Can you work these out from the model? Positions are in its coordinate system, mm. A direction names the side the tool comes from. Give positions to 0.01 mm unless a question says otherwise; leave off trailing zeros. Order: outer loops, then holes, each group sorted by start corner. A loop starts at its lowest first (then second) coordinate and runs counter-clockwise, first axis right, second up. Notation, with made-up numbers: (11, 82.25) - (54, 82.25) arc R24 ccw to (54, 94.25) - close; hole circle Ø4 at (55, 58). An arc over 180 degrees is marked (long way). Answer as a JSON object with one key per item and string values.
Autodesk Inventor part; units mm, degrees
ref_plane "YZ Plane" through (0, 0, 0) normal (1, 0, 0) x (0, 1, 0)
ref_plane "XZ Plane" through (0, 0, 0) normal (0, 1, 0) x (-1, 0, 0)
ref_plane "XY Plane" through (0, 0, 0) normal (0, 0, 1) x (1, 0, 0)
sketch "Sketch1" plane through (0, 0, 0) normal (0, 1, 0) x (-1, 0, 0)
  circle A0 centre (0, 0) radius 24.125
  arc A1 (-16.2075, 21.7505) -> (16.2075, 21.7505) centre (0, 0) ccw
  line L0 (15, 28) -> (-15, 28)
  line L1 (-15, 28) -> (-15, 25.1875)
  line L2 (15, 24.1561) -> (15, 28)
  line L3 (15, 28) -> (-15, 25.1875) construction
  line L4 (-15, 28) -> (15, 24.7857) construction
  line L5 (-15, 25.1875) -> (-15, 24.1561)
  arc A2 (15, 24.1561) -> (16.2075, 21.7505) centre (18, 24.1561) ccw
  arc A3 (-16.2075, 21.7505) -> (-15, 24.1561) centre (-18, 24.1561) ccw
  point P0 (-1, 26.5)
  point P1 (0, 26.3929)
  point P2 (15, 22.6001)
  point P3 (-15, 22.6001)
  dimension "d0" = 48.25
  dimension "d2" = 3
  dimension "d4" = 30
  dimension "d6" = 28
  dimension "d7" = 3
extrude "Extrusion1" add sketch "Sketch1" along normal blind 63.5
sketch "Sketch2" plane through (-15, 0, 28) normal (0, 0, 1) x (1, 0, 0)
  line L0 (30, 0) -> (30, 63.5)
  line L1 (0, 50.25) -> (30, 50.25)
  line L2 (30, 50.25) -> (30, 53.25)
  line L3 (30, 53.25) -> (0, 53.25)
  line L4 (0, 53.25) -> (0, 50.25)
  line L5 (0, 50.25) -> (30, 53.25) construction
  line L6 (30, 50.25) -> (0, 53.25) construction
  line L7 (0, 10.25) -> (30, 10.25)
  line L8 (30, 10.25) -> (30, 13.25)
  line L9 (30, 13.25) -> (0, 13.25)
  line L10 (0, 13.25) -> (0, 10.25)
  line L11 (0, 10.25) -> (30, 13.25) construction
  line L12 (30, 10.25) -> (0, 13.25) construction
  line L13 (0, 0) -> (0, 63.5)
  line L14 (0, 31.75) -> (30, 31.75) construction
  point P0 (15, 0)
  point P1 (15, 51.75)
  point P2 (15, 11.75)
  dimension "d10" = 3
  dimension "d11" = 3
  dimension "d12" = 40
  dimension "d13" = 20
  dimension "d34" = 30
  dimension "d35" = 30
extrude "Extrusion2" add sketch "Sketch2" along normal blind 35 contours L7 L10 L9 L0 | L1 L4 L3 L0
fillet "Fillet1" radius 14 4 edges at (-15, 51.75, 63) (15, 11.75, 63) (15, 51.75, 63) (-15, 11.75, 63)
sketch "Sketch3" plane through (-15, 53.25, 28) normal (0, 1, 0) x (1, 0, 0)
  arc A0 (0, -21) -> (30, -21) centre (16, -21) ccw
  point P0 (15, 28)
hole "Hole1" at (1, 53.25, 49) direction (0, -1, 0) diameter 9 end through all
fillet "Fillet2" radius 1 4 edges at (0, 53.25, 28) (0, 50.25, 28) (0, 13.25, 28) (0, 10.25, 28)
sketch "Sketch4" plane through (0, 0, 0) normal (0, 0, 1) x (1, 0, 0)
  line L0 (16.2075, 0) -> (16.2075, 63.5)
  line L1 (16.2075, 31.75) -> (-16.2075, 31.75)
  line L2 (-16.2075, 0) -> (-16.2075, 63.5)
  point P0 (0, 0)
  point P1 (0, 49.25)
  point P2 (0, 14.25)
  point P3 (0, 31.75)
  dimension "d25" = 17.5
  dimension "d26" = 17.5
hole "Hole2" at (0, 49.25, 0) at (0, 14.25, 0) direction (0, 0, -1) diameter 6.6 end through all
properties part number "Hanger_Clamp" material "Steel, Carbon"
Q1. If we section it at D-D, the plane z = 48: Please give me the cut outline in (x, y).
Recorded:
{"outline": "(-15, 10.25) - (-3.39, 10.25) - (-3.39, 13.25) - (-15, 13.25) - close; (-15, 50.25) - (-3.39, 50.25) - (-3.39, 53.25) - (-15, 53.25) - close; (5.39, 10.25) - (15, 10.25) - (15, 13.25) - (5.39, 13.25) - close; (5.39, 50.25) - (15, 50.25) - (15, 53.25) - (5.39, 53.25) - close"}
Q2. I'm going to push flat-ended pins straight in: pin 1 Ø15 at (x, y) = (-3.5, 23) entering from +Z; pin 2 Ø24 at (x, z) = (2.5, 50.5) entering from +Y; pin 3 Ø24 at (x, z) = (0.5, 46) entering from -Y. Where does each tip first touch, or does it pass through?
Recorded:
{"pin 1": "stops at z = 28", "pin 2": "stops at y = 53.25", "pin 3": "stops at y = 10.25"}
Q3. Which directions (+Z, -Z, +X, -X, +Y, -Y) give clear straight access to the entire face, cutting with the end or side of a thin tool? Please do faces 1 (the face through (15, 32, 27)), 2 (the face through (0, 10.25, 42)), 3 (the face through (0, 13.25, 42)), 4 (the face through (-3.27, 14.68, -25.53)).
Recorded:
{"face 1": "+Z, +X, +Y, -Y", "face 2": "+Z, +X, -X, -Y", "face 3": "+Z, +X, -X", "face 4": "-Z"}
Q4. If we section it at A-A, the plane z = 0: Please give me the cut outline in (x, y) (3 decimals), then the cut area to 3 significant figures.
Recorded:
{"outline": "(-27.125, 0) - (-24.125, 0) - (-24.125, 63.5) - (-27.125, 63.5) - close; (24.125, 0) - (27.125, 0) - (27.125, 63.5) - (24.125, 63.5) - close", "area": "381 mm^2"}
Q5. I need wall thicknesses on L1, parallel to Y at x = 0, z = -25; L2, parallel to Z at x = 1, y = 11; L3, parallel to X at y = 11.3, z = 49. Which ranges of each line are inside material? Lowest first, please.
Recorded:
{"L1": "y = 0 to 10.95, 17.55 to 45.95, 52.55 to 63.5", "L2": "z = -27.11 to -24.1, 24.1 to 44.5, 53.5 to 63", "L3": "x = -15 to -3.5, 5.5 to 15"}
Q6. We'd pull the mould along Z, two halves only. Please class faces 5 (the face through (-0.352, 51.729, 53.292)), 6 (the face through (0, 12, 63)), 7 (the face through (0, 53.25, 42)): released by +Z, released by -Z, zero draft, split by the parting line, or undercut.
Recorded:
{"face 5": "undercut", "face 6": "released by +Z", "face 7": "zero draft"}
Q7. If we section it at C-C, the plane x = -7: Please give me the cut outline in (y, z), then the cut area to 3 significant figures.
Recorded:
{"outline": "(0, -26.21) - (63.5, -26.21) - (63.5, -23.09) - (0, -23.09) - close; (0, 23.09) - (63.5, 23.09) - (63.5, 28) - (54.25, 28) arc R1 cw to (53.25, 29) - (53.25, 61.65) - (50.25, 61.65) - (50.25, 29) arc R1 cw to (49.25, 28) - (14.25, 28) arc R1 cw to (13.25, 29) - (13.25, 61.65) - (10.25, 61.65) - (10.25, 29) arc R1 cw to (9.25, 28) - (0, 28) - close", "area": "713 mm^2"}
